from build123d import *

# Parameters (mm, degrees)
SKETCH1_R           = 1.1
BOSS_EXTRUDE1_DEPTH = 4.8
SKETCH2_W           = 11.7
SKETCH2_H           = 6.188
SKETCH2_W_2         = 4.75
SKETCH2_H_2         = 3.4
CUT_EXTRUDE1_DEPTH  = 4.8
FILLET1_R           = 1


with BuildPart() as part:
    # Sketch1 → Boss-Extrude1 (new, symmetric)
    with BuildSketch(Plane.XY):
        with BuildLine():
            Line((-9.5, -2.5), (9.5, -2.5))
            Line((9.5, -2.5), (10.3, -2.5))
            ThreePointArc((10.3, -2.5), (11.148528137, -2.148528137), (11.5, -1.3))
            Line((11.5, -1.3), (11.5, -0.801473335))
            Line((11.5, -0.801473335), (11.5, 1.3))
            ThreePointArc((11.5, 1.3), (11.148528137, 2.148528137), (10.3, 2.5))
            Line((10.3, 2.5), (9.5, 2.5))
            Line((9.5, 2.5), (-9.5, 2.5))
            ThreePointArc((-9.5, 2.5), (-12, 0), (-9.5, -2.5))
        make_face()
        with Locations((-9.5, 0)):
            Circle(SKETCH1_R, mode=Mode.SUBTRACT)
        with Locations((9.5, 0)):
            Circle(SKETCH1_R, mode=Mode.SUBTRACT)
    extrude(amount=BOSS_EXTRUDE1_DEPTH, both=True)

    # Sketch2 → Cut-Extrude1 (cut, symmetric)
    with BuildSketch(Plane(origin=(0, 0, 0), x_dir=(1, 0, 0), z_dir=(0, 1, 0))):
        with Locations((2.85, 0)):
            Rectangle(SKETCH2_W, SKETCH2_H)
        with Locations((-9.625, 0)):
            Rectangle(SKETCH2_W_2, SKETCH2_H_2)
    extrude(amount=CUT_EXTRUDE1_DEPTH, both=True, mode=Mode.SUBTRACT)

    # Sketch6 → Revolve5 (revolve)
    with BuildSketch(Plane.XY):
        with BuildLine():
            Line((11.5, -1.24), (13.5, -1.24))
            add(Edge.make_bspline(
                [(13.5, -1.24), (14.590825895, -4.518170639), (18.155142557, -3.978926497), (21.719459219, -3.439682355), (21.696199677, 0)],
                knots=[3.442238671, 3.442238671, 3.442238671, 4.862711989, 4.862711989, 6.283185307, 6.283185307, 6.283185307], degree=2, weights=[1, 0.758207592, 1, 0.758207592, 1]))
            Line((21.696199677, 0), (11.5, 0))
            Line((11.5, 0), (11.5, -1.24))
        make_face()
    revolve(axis=Axis((11.5, 0, 0), (1, 0, 0)))

    # Fillet1
    fillet1_edges = [part.edges().sort_by_distance(p)[0] for p in [
        (-7.25, 0, 1.7),
        (-7.25, 0, -1.7),
    ]]
    fillet(fillet1_edges, radius=FILLET1_R)


solid = part.part
The listing builds one solid part. Answer for the finished solid, in the listing's coordinates (mm). A direction names the side the tool comes from. Give positions to 0.01 mm unless a question says otherwise; leave off trailing zeros. Write each loop counter-clockwise with the first axis right and the second up, starting at its lowest first coordinate (ties: lowest second). Pieces come first, ordered by that corner, then holes.
Item 1: Determine the mould class of faces 1 (the flat face through (0, 0, 4.8)), 2 (the cylindrical face through (-7.551, -0.035, -1.415)), 3 (the cylindrical face through (11.158, 2.139, 0.067)) for opening direction X: released by +X, released by -X, zero draft, split by the parting line, or undercut.
Item 2: Which of the six approach directions +Z, -Z, +X, -X, +Y, -Y give full straight-line access (tool end or side, diameter ignored) to faces 4 (the cylindrical face through (12.51, 0.27, 1.21)), 5 (the flat face through (-11, 1, -1.7)), 6 (the flat face through (8.7, 2, 0)), 7 (the flat face through (0.3, -2.5, 3.3))?
Item 3: Section A-A, the plane x = 9.5 is taken. Write down the section's boundary in (y, z).
Item 4: Find the intervals of material crossed by line 1 along X through (y, z) = (0, 4.15); line 2 along Y through (x, z) = (-9.5, 2.4); line 3 along X through (y, z) = (0, -3), in increasing order.
Item 5: Section B-B, the plane z = 2.25 is taken. Count the separate pieces of the cut face and the enclosed holes in it, plus the area to 3 significant figures.
Item 6: Flat-ended cylindrical pins translate along their axes: P1, Ø1, axis at x = 14.5, z = 0.5, coming from the +Y side; P2, Ø1.5, axis at x = 17.5, y = -1, coming from the -Z side; P3, Ø1.1, axis at x = -9.5, y = -0.5, coming from the -Z side; P4, Ø0.5, axis at y = -2, z = 0, coming from the -X side. Find the tip coordinate at first contact, or state that the pin passes through.
Completed:
1. face 1: zero draft
1. face 2: released by -X
1. face 3: undercut
2. face 4: none
2. face 5: -X, +Y, -Y
2. face 6: +Y, -Y
2. face 7: +Z, -Z, -X, -Y
3. outline: (-2.5, -4.8) - (-1.1, -4.8) - (-1.1, 4.8) - (-2.5, 4.8) - close; (1.1, -4.8) - (2.5, -4.8) - (2.5, 4.8) - (1.1, 4.8) - close
4. line 1: x = -12 to -10.6, -8.4 to 8.4, 10.6 to 11.5
4. line 2: y = -2.5 to -1.1, 1.1 to 2.5
4. line 3: x = -12 to -10.6, -8.4 to -3, 10.6 to 11.5, 14.69 to 20.31
5. separate pieces: 3
5. enclosed holes: 1
5. area: 85.1 mm2
6. P1: stops at y = 3.21
6. P2: stops at z = -4.02
6. P3: passes through
6. P4: stops at x = -7.25
